Answer from the drawing. Dimensions are ordinates in mm from the lowest x, y and z of the part. A direction names the side the tool comes from. Coordinates: 2 decimals unless noted, no trailing zeros. Loops run counter-clockwise (first coordinate to the right, second up) from the corner with the lowest first, then second, coordinate; pieces in that order, holes last. Notation, with made-up numbers: (70.25, 39.5) -> (105.25, 39.5) arc R16 ccw to (105.25, 67.5) -> close; hole circle Ø6 at (79.25, 1). An arc over 180 degrees is marked (long way). Use a Markdown table: item, result.
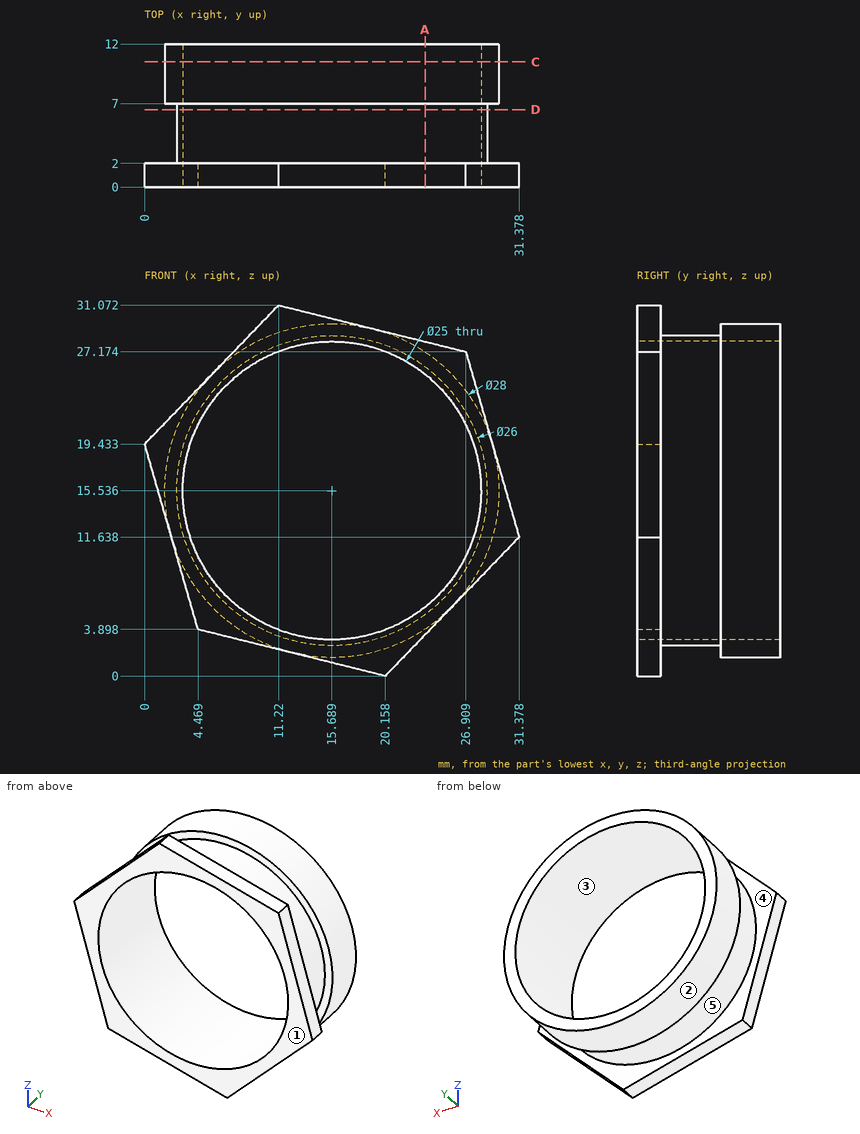
Q1. Determine the mould class of the marked faces 3, 4 and 5 for opening direction Z: pulls with the +Z half, pulls with the -Z half, needs draft (parallel to the pull), parting line crosses it, or undercut.
Solved:
| item | result |
|---|---|
| face 3 | undercut |
| face 4 | needs draft |
| face 5 | parting line crosses it |
Q2. For the marked faces 1 and 2, determine the directions among +Z, -Z, +X, -X, +Y, -Y from which every point of the face is accessible in a straight line to the end or side of a thin tool.
Solved:
| item | result |
|---|---|
| face 1 | +Z, -Z, +X, -X, -Y |
| face 2 | +Y |
Q3. Section A-A on x = 23.5 is taken. Determine the outline of the cut face in (y, z) (1 decimal).
Solved:
| item | result |
|---|---|
| outline | (0, 3.5) -> (2, 3.5) -> (2, 5.1) -> (7, 5.1) -> (7, 3.9) -> (12, 3.9) -> (12, 5.8) -> (0, 5.8) -> close; (0, 25.3) -> (12, 25.3) -> (12, 27.2) -> (7, 27.2) -> (7, 25.9) -> (2, 25.9) -> (2, 28) -> (0, 28) -> close |
Q4. Given pin 1 Ø6 at (y, z) = (8.5, 7) entering from +X; pin 2 Ø1 at (x, y) = (10, 7.5) entering from +Z, each flat-ended and moving along its own axis, determine where each tip first touches the part or whether it passes through.
Solved:
| item | result |
|---|---|
| pin 1 | x = 28.55 |
| pin 2 | z = 28.54 |
Q5. Section C-C on y = 10.5 is taken. Determine the outline of the cut face in (x, z) (1 decimal).
Solved:
| item | result |
|---|---|
| outline | circle Ø28 at (15.7, 15.5); hole circle Ø25 at (15.7, 15.5) |
Q6. Consider line 1 (Y direction, x = 29, z = 11.5); line 2 (Z direction, x = 26, y = 10.75) (1 decimal); line 3 (X direction, y = 3.5, z = 7) (1 decimal). Determine where each line is inside the solid, lowest interval first. Write a range as [from, to].
Solved:
| item | result |
|---|---|
| line 1 | [0, 2], [7, 12] |
| line 2 | [6.1, 8.5], [22.6, 25] |
| line 3 | [5.9, 6.6], [24.8, 25.5] |
Q7. Section D-D on y = 6.5 is taken. Determine the outline of the cut face in (x, z) (1 decimal).
Solved:
| item | result |
|---|---|
| outline | circle Ø26 at (15.7, 15.5); hole circle Ø25 at (15.7, 15.5) |
